Geometry: final body of the model. Coordinates: model frame, mm. Face numbers are marked on the shaded views. Give positions to 0.01 mm unless a question says otherwise; leave off trailing zeros. Order: outer loops, then holes, each group sorted by start corner. A loop starts at its lowest first (then second) coordinate and runs counter-clockwise, first axis right, second up. Notation, with made-up numbers: (-15.75, -2) -> (29.25, -2) arc R20 ccw to (29.25, 21) -> close; hole circle Ø9 at (-38, 58.5). An arc over 180 degrees is marked (long way). One line per question, with ' | ' between items.
from build123d import *

# Parameters (mm, degrees)
EXTRUDE_1_DEPTH            = 48
CUT_EXTRUDE_2_REACH        = 96.508
CUT_EXTRUDE_2_START_RADIUS = 70
CUT_EXTRUDE_2_END_RADIUS   = 70
SKETCH_3_W                 = 58.404028666
SKETCH_3_H                 = 6
EXTRUDE_2_DEPTH            = 13
CUT_EXTRUDE_3_DEPTH        = 140.034418617
CUT_EXTRUDE_3_DEPTH_BACK   = 140.034418617
SKETCH_4_W                 = 25
SKETCH_4_H                 = 38
SKETCH_4_W_2               = 40
SKETCH_4_H_2               = 25
CHAMFER_1_SIZE             = 5
CHAMFER_1_SIZE2            = 3.813196151
SKETCH_6_R                 = 6.5
CUT_EXTRUDE_4_DEPTH        = 2
SKETCH_7_R                 = 1.5
CUT_EXTRUDE_5_DEPTH        = 60
SKETCH_8_W                 = 9
SKETCH_8_H                 = 9
CUT_EXTRUDE_6_DEPTH        = 11
CUT_EXTRUDE_8_REACH        = 137.533
SKETCH_10_R                = 1
CUT_EXTRUDE_9_REACH        = 105.034
CUT_EXTRUDE_9_END_RADIUS   = 70
SKETCH_11_R                = 0.75
SKETCH_12_W                = 20
SKETCH_12_H                = 3
CUT_EXTRUDE_10_DEPTH       = 11
SKETCH_13_W                = 3.868283576
SKETCH_13_H                = 1.5
CUT_EXTRUDE_11_DEPTH       = 4
CUT_EXTRUDE_12_REACH       = 137.476
SKETCH_15_OUTSIDE_W        = 122.502
SKETCH_15_OUTSIDE_H        = 162.955
SKETCH_15_OUTSIDE_W_2      = 109.971714071
SKETCH_15_OUTSIDE_H_2      = 49.254432198
CUT_EXTRUDE_13_DEPTH       = 10


with BuildPart() as part:
    # 草图1 → 凸台-拉伸1 (new body)
    with BuildSketch(Plane(origin=(0, 0, 0), x_dir=(1, 0, 0), z_dir=(0, 1, 0))):
        with BuildLine():
            ThreePointArc((-9.396926208, -7.075874358), (-5.735764364, -11.847193368), (0, -13.655672925))
            Line((0, -13.655672925), (0, -5))
            ThreePointArc((0, -5), (-5, 0), (0, 5))
            Line((0, 5), (0, 70))
            ThreePointArc((0, 70), (-17.673593853, 67.732149533), (-34.202014333, 61.075545152))
            Line((-34.202014333, 61.075545152), (-9.396926208, -7.075874358))
        make_face()
        with BuildLine():
            Line((0, -5), (0, -13.655672925))
            ThreePointArc((0, -13.655672925), (5.735764364, -11.847193368), (9.396926208, -7.075874358))
            Line((9.396926208, -7.075874358), (34.202014333, 61.075545152))
            ThreePointArc((34.202014333, 61.075545152), (17.673593853, 67.732149533), (0, 70))
            Line((0, 70), (0, 5))
            ThreePointArc((0, 5), (3.535533906, 3.535533906), (5, 0))
            ThreePointArc((5, 0), (3.535533906, -3.535533906), (0, -5))
        make_face()
    extrude(amount=EXTRUDE_1_DEPTH)

    # 切除-拉伸2: from a cylinder face, 96.508 long prism both ways, kept between that surface and its translate by the depth
    cut_extrude_2_start = Plane(origin=(0, 5, 0), z_dir=(0, -1, 0)) * Cylinder(CUT_EXTRUDE_2_START_RADIUS, 334.016, mode=Mode.PRIVATE)
    cut_extrude_2_end = Plane(origin=(0, 5, 3), z_dir=(0, -1, 0)) * Cylinder(CUT_EXTRUDE_2_END_RADIUS, 334.016, mode=Mode.PRIVATE)
    # 草图3 → 切除-拉伸2 (cut, from a surface)
    with BuildSketch(Plane.XY, mode=Mode.PRIVATE) as cut_extrude_2_sk1:
        with Locations((3, 5)):
            Rectangle(SKETCH_3_W, SKETCH_3_H)
    cut_extrude_2_tool1 = extrude(cut_extrude_2_sk1.sketch, amount=CUT_EXTRUDE_2_REACH, both=True, mode=Mode.PRIVATE)
    add(((cut_extrude_2_tool1 & cut_extrude_2_start) - cut_extrude_2_end).solids().sort_by_distance((3, 5, -62.032204))[0], mode=Mode.SUBTRACT)

    # 草图2 → 凸台-拉伸2 (add)
    with BuildSketch(Plane(origin=(0, 48, 0), x_dir=(1, 0, 0), z_dir=(0, 1, 0))):
        Polygon((24.252642572, 33.739870901), (55.034455471, 118.312206771), (20.125623779, 80.877067961), (5.458790156, 40.580273767), align=None)
    extrude(amount=-EXTRUDE_2_DEPTH)

    # 草图4 → 切除-拉伸3 (cut, two sides: drawn at the far end of the back side and taken through both)
    with BuildSketch(Plane(origin=(0, 0, 0), x_dir=(0, 0, -1), z_dir=(1, 0, 0)).offset(-CUT_EXTRUDE_3_DEPTH_BACK)):
        with Locations((-1.155672925, 29)):
            Rectangle(SKETCH_4_W, SKETCH_4_H)
        with Locations((50.466884927, 22.5)):
            Rectangle(SKETCH_4_W_2, SKETCH_4_H_2)
    extrude(amount=CUT_EXTRUDE_3_DEPTH + CUT_EXTRUDE_3_DEPTH_BACK, mode=Mode.SUBTRACT)

    # 倒角1
    chamfer_1_edges = [part.edges().sort_by_distance(p)[0] for p in [
        (55.034455471, 41.5, -118.312206771),
    ]]
    chamfer_1_side = [part.faces().sort_by_distance(p)[0] for p in [
        (37.580039625, 41.5, -99.594637366),
    ]]
    chamfer(chamfer_1_edges, length=CHAMFER_1_SIZE, length2=CHAMFER_1_SIZE2, reference=chamfer_1_side[0])

    # 草图6 → 切除-拉伸4 (cut)
    with BuildSketch(Plane.XZ):
        with Locations(Location((0, 0, 0), (0, 0, 270))):
            Circle(SKETCH_6_R)
    extrude(amount=-CUT_EXTRUDE_4_DEPTH, mode=Mode.SUBTRACT)

    # 草图7 → 切除-拉伸5 (cut)
    with BuildSketch(Plane.XY):
        with Locations((-30.202014333, 5)):
            Circle(SKETCH_7_R)
    extrude(amount=-CUT_EXTRUDE_5_DEPTH, mode=Mode.SUBTRACT)

    # 草图8 → 切除-拉伸6 (cut)
    with BuildSketch(Plane(origin=(0, 10, 0), x_dir=(1, 0, 0), z_dir=(0, 1, 0))):
        with Locations((-30.258231885, 50.240091929)):
            Rectangle(SKETCH_8_W, SKETCH_8_H)
    extrude(amount=-CUT_EXTRUDE_6_DEPTH, mode=Mode.SUBTRACT)

    # 切除-拉伸8: up to this plane
    cut_extrude_8_end = Plane(origin=(32.202014333, 48, -62.153280468), z_dir=(-1, 0, 0))
    # 草图10 → 切除-拉伸8 (cut, up to the surface)
    with BuildSketch(Plane(origin=(10.571836839, 0, 3.847833931), x_dir=(0.34202014332566283, 0, -0.9396926207859106), z_dir=(0.9396926207859106, 0, 0.34202014332566283)), mode=Mode.PRIVATE) as cut_extrude_8_sk1:
        with Locations((67.590016934, 5)):
            Circle(SKETCH_10_R)
    cut_extrude_8_tool1 = split(extrude(cut_extrude_8_sk1.sketch, amount=-CUT_EXTRUDE_8_REACH, mode=Mode.PRIVATE), bisect_by=cut_extrude_8_end, keep=Keep.BOTH, mode=Mode.PRIVATE)
    add(cut_extrude_8_tool1.solids().sort_by_distance((33.688984, 5, -59.666006))[0], mode=Mode.SUBTRACT)

    # 切除-拉伸9: up to this cylinder (the profile starts inside it)
    cut_extrude_9_end = Plane(origin=(0, 5, 0), z_dir=(0, -1, 0)) * Cylinder(CUT_EXTRUDE_9_END_RADIUS, 351.068, mode=Mode.PRIVATE)
    # 草图11 → 切除-拉伸9 (cut, up to the surface)
    with BuildSketch(Plane.XY.offset(-60), mode=Mode.PRIVATE) as cut_extrude_9_sk1:
        with Locations((-30.202014333, 5)):
            Circle(SKETCH_11_R)
    cut_extrude_9_tool1 = extrude(cut_extrude_9_sk1.sketch, amount=-CUT_EXTRUDE_9_REACH, mode=Mode.PRIVATE) & cut_extrude_9_end
    add(cut_extrude_9_tool1.solids().sort_by_distance((-30.202014, 5, -60))[0], mode=Mode.SUBTRACT)

    # 草图12 → 切除-拉伸10 (cut)
    with BuildSketch(Plane(origin=(0, 10, 0), x_dir=(1, 0, 0), z_dir=(0, 1, 0))):
        with Locations((8.346963974, 51.411545488)):
            Rectangle(SKETCH_12_W, SKETCH_12_H)
    extrude(amount=-CUT_EXTRUDE_10_DEPTH, mode=Mode.SUBTRACT)

    # 草图13 → 切除-拉伸11 (cut)
    with BuildSketch(Plane(origin=(0, 10, 0), x_dir=(1, 0, 0), z_dir=(0, 1, 0))):
        with Locations((29.542762739, 51.411545488)):
            Rectangle(SKETCH_13_W, SKETCH_13_H)
    extrude(amount=-CUT_EXTRUDE_11_DEPTH, mode=Mode.SUBTRACT)

    # 草图14 → 切除-拉伸12 (cut, up to next)
    with BuildSketch(Plane(origin=(0, 48, 0), x_dir=(1, 0, 0), z_dir=(0, 1, 0)), mode=Mode.PRIVATE) as cut_extrude_12_sk1:
        Polygon((49.766128767, 108.223290792), (49.034775066, 108.905289152), (40.168796385, 99.397691031), (40.900150086, 98.715692671), align=None)
    cut_extrude_12_tool1 = extrude(cut_extrude_12_sk1.sketch, amount=-CUT_EXTRUDE_12_REACH, mode=Mode.PRIVATE) & part.part
    add(cut_extrude_12_tool1.solids().sort_by_distance((44.967463, 48, -103.810491))[0], mode=Mode.SUBTRACT)

    # 草图15 outside → 切除-拉伸13 (cut)
    with BuildSketch(Plane(origin=(0, 10, 0), x_dir=(1, 0, 0), z_dir=(0, 1, 0))):
        with Locations((9.764, 50.5365)):
            Rectangle(SKETCH_15_OUTSIDE_W, SKETCH_15_OUTSIDE_H)
        with Locations((3.943147272, 55.094101026)):
            Rectangle(SKETCH_15_OUTSIDE_W_2, SKETCH_15_OUTSIDE_H_2, mode=Mode.SUBTRACT)
    extrude(amount=-CUT_EXTRUDE_13_DEPTH, mode=Mode.SUBTRACT)


with BuildPart() as body_2:
    # of the pieces the cut leaves, the one that is kept (cut_extrude_13_keep)
    add(part.part.solids().sort_by_distance((23.0613731, 0, -30.466884927))[0])


solid = body_2.part
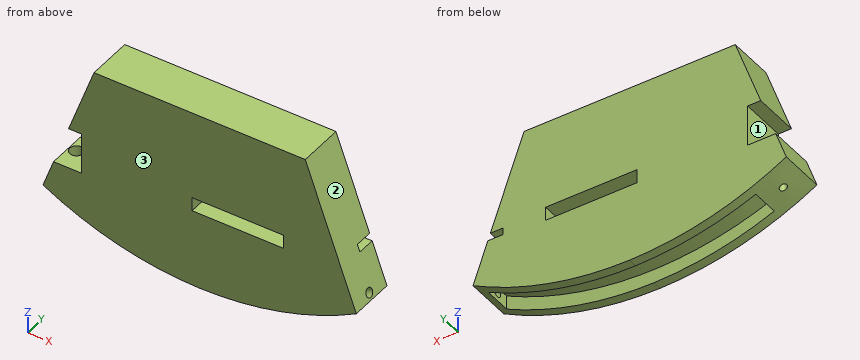
1) Material intervals for probe 1 along X at (y, z) = (5, -61.8); probe 2 along Y at (x, z) = (-2, -67); probe 3 along Z at (x, y) = (16, 0.75), sorted ascending. Write a range as from..to.
Check result:
probe 1: x = -32.87..-30.95, -29.45..26.48, 32.2..32.87 | probe 2: y = 0..2, 8..10 | probe 3: z = -68.15..-52.91, -49.91..-30.47
2) Pull-direction query (Z, two-part tool) for the marked faces 1, 2 and 3; classes: +Z half, -Z half, draft (parallel to the pull), parting line (faces both ways), or undercut.
Check result:
face 1: undercut | face 2: +Z half | face 3: draft
3) Section A-A on x = 3. Return loops of the section in (y, z).
Check result:
outline: (0, -69.94) -> (2, -69.94) -> (2, -66.94) -> (8, -66.94) -> (8, -69.94) -> (10, -69.94) -> (10, -52.91) -> (0, -52.91) -> close; (0, -49.91) -> (10, -49.91) -> (10, -30.47) -> (0, -30.47) -> close
4) Section B-B on x = -12.5. Return loops of the section in (y, z), plus the area to 3 significant figures.
Check result:
outline: (0, -68.87) -> (2, -68.87) -> (2, -65.87) -> (8, -65.87) -> (8, -68.87) -> (10, -68.87) -> (10, -30.47) -> (0, -30.47) -> close | area: 366 mm^2
5) Section C-C on z = -66. Return loops of the section in (x, y), plus the area to 3 significant figures.
Check result:
outline: (-23.32, 0) -> (23.32, 0) -> (23.32, 2) -> (11.79, 2) -> (11.79, 8) -> (23.32, 8) -> (23.32, 10) -> (-23.32, 10) -> (-23.32, 8) -> (-11.79, 8) -> (-11.79, 2) -> (-23.32, 2) -> close | area: 328 mm^2
6) Contact query for flat-ended pins moving along their axis: pin 1 Ø1.5 at (y, z) = (1, -55) entering from -X; pin 2 Ø1.5 at (y, z) = (6, -62.5) entering from +X; pin 3 Ø0.5 at (x, z) = (30, -51) entering from +Y; pin 4 Ø5.5 at (x, z) = (1, -62) entering from -Y. Output: stop coordinate, or through.
Check result:
pin 1: stops at x = -32.26 | pin 2: stops at x = 32.97 | pin 3: stops at y = 6 | pin 4: stops at y = 0
7) Section D-D on z = -34.5. Return loops of the section in (x, y).
Check result:
outline: (-24.53, 0) -> (24.53, 0) -> (24.53, 10) -> (-24.53, 10) -> close
